Autodesk Inventor part; units mm, degrees
ref_plane "YZ Plane" through (0, 0, 0) normal (1, 0, 0) x (0, 1, 0)
ref_plane "XZ Plane" through (0, 0, 0) normal (0, 1, 0) x (-1, 0, 0)
ref_plane "XY Plane" through (0, 0, 0) normal (0, 0, 1) x (1, 0, 0)
sketch "Sketch1" plane through (0, 0, 0) normal (0, 0, 1) x (1, 0, 0)
  line L0 (0, 0) -> (56, 0) construction
  line L1 (56, 0) -> (56, 56) construction
  line L2 (56, 56) -> (0, 56) construction
  line L3 (0, 56) -> (0, 0) construction
  line L4 (0, 47) -> (9, 47)
  line L5 (9, 47) -> (9, 56)
  line L6 (9, 56) -> (47, 56)
  line L7 (47, 56) -> (47, 47)
  line L8 (47, 47) -> (56, 47)
  line L9 (56, 47) -> (56, 9)
  line L10 (56, 9) -> (47, 9)
  line L11 (47, 9) -> (47, 0)
  line L12 (47, 0) -> (9, 0)
  line L13 (9, 0) -> (9, 9)
  line L14 (9, 9) -> (0, 9)
  line L15 (0, 9) -> (0, 47)
  dimension "d0" = 56
  dimension "d1" = 38
extrude "Extrusion1" add sketch "Sketch1" along normal blind 48
sketch "Sketch2" plane through (0, 0, 48) normal (0, 0, 1) x (1, 0, 0)
  line L0 (9, 47) -> (0, 47)
  line L1 (0, 47) -> (0, 9)
  line L2 (0, 9) -> (9, 9)
  line L3 (9, 9) -> (9, 0)
  line L4 (9, 0) -> (47, 0)
  line L5 (47, 0) -> (47, 9)
  line L6 (47, 9) -> (56, 9)
  line L7 (56, 9) -> (56, 47)
  line L8 (56, 47) -> (47, 47)
  line L9 (47, 47) -> (47, 56)
  line L10 (47, 56) -> (9, 56)
  line L11 (9, 56) -> (9, 47)
  line L12 (9, 47) -> (0, 47)
  line L13 (0, 47) -> (0, 56)
  line L14 (0, 56) -> (9, 56)
  line L15 (9, 56) -> (9, 47)
  line L16 (47, 47) -> (56, 47)
  line L17 (47, 47) -> (56, 47)
  line L18 (56, 47) -> (56, 56)
  line L19 (56, 56) -> (47, 56)
  line L20 (47, 56) -> (47, 47)
  line L21 (47, 9) -> (47, 0)
  line L22 (47, 9) -> (56, 9)
  line L23 (56, 9) -> (56, 0)
  line L24 (56, 0) -> (47, 0)
  line L25 (47, 0) -> (47, 9)
  line L26 (47, 0) -> (9, 0)
  line L27 (9, 9) -> (0, 9)
  line L28 (9, 0) -> (0, 0)
  line L29 (0, 0) -> (0, 9)
  line L30 (0, 9) -> (9, 9)
  line L31 (9, 9) -> (9, 0)
  line L32 (47, 9) -> (56, 9)
  line L33 (47, 0) -> (47, 9)
  line L34 (47, 47) -> (47, 56)
  circle A0 centre (4.5, 51.5) radius 2.5
  circle A1 centre (51.5, 51.5) radius 2.5
  circle A2 centre (51.5, 4.5) radius 2.5
  circle A3 centre (4.5, 4.5) radius 2.5
  line L35 (4.5, 51.5) -> (51.5, 51.5) construction
  line L36 (51.5, 51.5) -> (51.5, 4.5) construction
  line L37 (51.5, 4.5) -> (4.5, 4.5) construction
  line L38 (4.5, 4.5) -> (4.5, 51.5) construction
  line L39 (0, 56) -> (56, 0) construction
  line L40 (47, 47) -> (56, 56) construction
  line L41 (28, 51.5) -> (28, 28) construction
  line L42 (28, 28) -> (4.5, 28) construction
  arc A4 (4.5, 56) -> (0, 51.5) centre (4.5, 51.5) ccw
  arc A5 (56, 51.5) -> (51.5, 56) centre (51.5, 51.5) ccw
  arc A6 (0, 4.5) -> (4.5, 0) centre (4.5, 4.5) ccw
  arc A7 (51.5, 0) -> (56, 4.5) centre (51.5, 4.5) ccw
  dimension "d4" = 5
  dimension "d5" = 47
extrude "Extrusion2" add sketch "Sketch2" along normal blind 4.8 contours L11 L10 L9 L8 L7 L6 L5 L4 L3 L2 L1 L0 | L0 L13 A4 L14 L11 | L2 L3 L28 A6 L29 | L19 A5 L18 L8 L9 | L5 L6 L23 A7 L24
sketch "Sketch3" plane through (0, 0, 52.8) normal (0, 0, 1) x (1, 0, 0)
  circle A0 centre (28, 28) radius 19
  circle A1 centre (4.5, 4.5) radius 2.5 construction
  circle A2 centre (51.5, 51.5) radius 2.5 construction
  line L0 (4.5, 4.5) -> (51.5, 51.5) construction
  point P0 (0, 0)
  dimension "d8" = 38
extrude "Extrusion3" add sketch "Sketch3" along normal blind 1.5
sketch "Sketch4" plane through (28, 28, 54.3) normal (0, 0, 1) x (1, 0, 0)
  circle A0 centre (0, 0) radius 3.15
  point P0 (-28, -28)
  dimension "d11" = 6.3
extrude "Extrusion4" add sketch "Sketch4" along normal blind 6.6
sketch "Sketch5" plane through (28, 28, 60.9) normal (0, 0, 1) x (1, 0, 0)
  circle A0 centre (0, 0) radius 3.15
  line L0 (-2.4739, -1.95) -> (2.4739, -1.95)
  circle A1 centre (0, 0) radius 3.15
  point P0 (-28, -28)
  dimension "d14" = 5.1
extrude "Extrusion5" add sketch "Sketch5" along normal blind 17 contours A0 L0 picked at (0.6783, 0.1866)
properties part number "Big Chungus Motor"
Geometry: final body of the model. Coordinates: model frame, mm. A direction names the side the tool comes from. Coordinates: 2 decimals unless noted, no trailing zeros. Loops run counter-clockwise (first coordinate to the right, second up) from the corner with the lowest first, then second, coordinate; pieces in that order, holes last. Notation, with made-up numbers: (52, 88.25) -> (90, 88.25) arc R24 ccw to (90, 103.25) -> close; hole circle Ø6 at (2, 36.5). An arc over 180 degrees is marked (long way). Use a Markdown table: item, result. Add a question column.
(1) Line query: line 1 along Y through (x, z) = (4.5, 51.6); line 2 along X through (y, z) = (51, 50). Output: solid intervals per line, ascending.
(2) Section query C-C, the plane z = 39. Return loops of the section in (x, y), plus the area to 3 significant figures.
(3) Pin query (flat end, axial travel): pin 1 Ø6.5 at (x, y) = (51.5, 51.5) entering from -Z; pin 2 Ø2.5 at (y, z) = (6, 20) entering from -X; pin 3 Ø0.6 at (x, y) = (28.5, 25.5) entering from +Z. Return the tip coordinate at first contact, or that it passes through.
(4) Section query D-D, the plane y = 34.5. Return loops of the section in (x, z), plus the area to 3 significant figures.
(5) Mould query, pull axis X, two halves, no side actions, for faces 6 (the cylindrical face through (1.283, 54.647, 50.366)), 7 (the cylindrical face through (53.81, 52.46, 50.37)), 8 (the flat face through (28, 56, 26)). Classes: pulls with the +X half, pulls with the -X half, needs draft (parallel to the pull), parting line crosses it, or undercut.
(6) Access query for faces 1 (the cylindrical face through (53.81, 5.46, 50.37)), 2 (the flat face through (49, 50, 48)), 3 (the flat face through (4, 47, 24)), 4 (the flat face through (6, 7, 48)), 5 (the flat face through (21, 47, 52.8)). Directions: +Z, -Z, +X, -X, +Y, -Y. A direction counts if a zero-diameter tool reaches every point of the face in a straight line with its end or side. Return the directions, or none.
(7) Section query B-B, the plane x = 28. Return loops of the section in (y, z), plus the area to 3 significant figures.
(8) Section query A-A, the plane y = 50. Return loops of the section in (x, z), plus the area to 3 significant figures.
Answer:
| question | item | result |
|---|---|---|
| 1 | line 1 | y = 0 to 2, 7 to 49, 54 to 56 |
| 1 | line 2 | x = 0 to 2.05, 6.95 to 49.05, 53.95 to 56 |
| 2 | outline | (0, 9) -> (9, 9) -> (9, 0) -> (47, 0) -> (47, 9) -> (56, 9) -> (56, 47) -> (47, 47) -> (47, 56) -> (9, 56) -> (9, 47) -> (0, 47) -> close |
| 2 | area | 2,810 mm^2 |
| 3 | pin 1 | stops at z = 48 |
| 3 | pin 2 | stops at x = 9 |
| 3 | pin 3 | stops at z = 60.9 |
| 4 | outline | (0, 0) -> (56, 0) -> (56, 52.8) -> (45.85, 52.8) -> (45.85, 54.3) -> (10.15, 54.3) -> (10.15, 52.8) -> (0, 52.8) -> close |
| 4 | area | 3,010 mm^2 |
| 5 | face 6 | pulls with the -X half |
| 5 | face 7 | undercut |
| 5 | face 8 | needs draft |
| 6 | face 1 | +Z, -Z |
| 6 | face 2 | -Z, +X, +Y |
| 6 | face 3 | -Z, -X, +Y |
| 6 | face 4 | -Z, -X, -Y |
| 6 | face 5 | +Z |
| 7 | outline | (0, 0) -> (56, 0) -> (56, 52.8) -> (47, 52.8) -> (47, 54.3) -> (31.15, 54.3) -> (31.15, 77.9) -> (26.05, 77.9) -> (26.05, 60.9) -> (24.85, 60.9) -> (24.85, 54.3) -> (9, 54.3) -> (9, 52.8) -> (0, 52.8) -> close |
| 7 | area | 3,140 mm^2 |
| 8 | outline | (0, 48) -> (2.5, 48) -> (2.5, 52.8) -> (0, 52.8) -> close; (6.5, 48) -> (9, 48) -> (9, 0) -> (47, 0) -> (47, 48) -> (49.5, 48) -> (49.5, 52.8) -> (6.5, 52.8) -> close; (53.5, 48) -> (56, 48) -> (56, 52.8) -> (53.5, 52.8) -> close |
| 8 | area | 2,050 mm^2 |
